```python
from build123d import *

# Parameters (mm, degrees)
SKETCH1_W                                            = 35
SKETCH1_H                                            = 38
BOSS_EXTRUDE1_DEPTH                                  = 4
M3_CLEARANCE_HOLE1_D                                 = 3.4
SKETCH4_R                                            = 11.05
CUT_EXTRUDE1_DEPTH                                   = 5
M3_CLEARANCE_HOLE2_D                                 = 3.4
CSK_FOR_M3_HEX_SOCKET_COUNTERSUNK_CAP_SC_D           = 3.4
CSK_FOR_M3_HEX_SOCKET_COUNTERSUNK_CAP_SC_CSINK_D     = 6.72
CSK_FOR_M3_HEX_SOCKET_COUNTERSUNK_CAP_SC_CSINK_ANGLE = 90
CSK_FOR_M3_HEX_SOCKET_COUNTERSUNK_CA_2_D             = 3.4
CSK_FOR_M3_HEX_SOCKET_COUNTERSUNK_CA_2_CSINK_D       = 6.72
CSK_FOR_M3_HEX_SOCKET_COUNTERSUNK_CA_2_CSINK_ANGLE   = 90


with BuildPart() as part:
    # Sketch1 → Boss-Extrude1 (new body)
    with BuildSketch(Plane(origin=(0, 0, 0), x_dir=(1, 0, 0), z_dir=(0, 1, 0))):
        Rectangle(SKETCH1_W, SKETCH1_H)
    extrude(amount=BOSS_EXTRUDE1_DEPTH)

    # M3 Clearance Hole1 (through all)
    with Locations(Plane(origin=(0, 0, 0), x_dir=(-1, 0, 0), z_dir=(0, -1, 0))):
        with Locations((-11.5, -13.5), (-11.5, 9.5), (11.5, 9.5), (11.5, -13.5)):
            Hole(M3_CLEARANCE_HOLE1_D / 2)

    # Sketch4 → Cut-Extrude1 (cut, through all)
    with BuildSketch(Plane(origin=(0, 4, 0), x_dir=(1, 0, 0), z_dir=(0, 1, 0))):
        with Locations((0, 1.5)):
            Circle(SKETCH4_R)
    extrude(amount=-CUT_EXTRUDE1_DEPTH, mode=Mode.SUBTRACT)

    # M3 Clearance Hole2 (through all)
    with Locations(Plane(origin=(0, 4, 0), x_dir=(1, 0, 0), z_dir=(0, 1, 0))):
        with Locations((-13, 14.5), (13, 14.5), (-13, -11.5), (13, -11.5)):
            Hole(M3_CLEARANCE_HOLE2_D / 2)

    # CSK for M3 Hex Socket Countersunk Cap Sc (through all)
    with Locations(Plane(origin=(0, 0, 0), x_dir=(-1, 0, 0), z_dir=(0, -1, 0))):
        with Locations((-13, 14.5), (13, 14.5)):
            CounterSinkHole(CSK_FOR_M3_HEX_SOCKET_COUNTERSUNK_CAP_SC_D / 2, CSK_FOR_M3_HEX_SOCKET_COUNTERSUNK_CAP_SC_CSINK_D / 2, counter_sink_angle=CSK_FOR_M3_HEX_SOCKET_COUNTERSUNK_CAP_SC_CSINK_ANGLE)

    # CSK for M3 Hex Socket Countersunk Ca 2 (through all)
    with Locations(Plane(origin=(0, 4, 0), x_dir=(1, 0, 0), z_dir=(0, 1, 0))):
        with Locations((11.5, 9.5), (-11.093205122, 9.5)):
            CounterSinkHole(CSK_FOR_M3_HEX_SOCKET_COUNTERSUNK_CA_2_D / 2, CSK_FOR_M3_HEX_SOCKET_COUNTERSUNK_CA_2_CSINK_D / 2, counter_sink_angle=CSK_FOR_M3_HEX_SOCKET_COUNTERSUNK_CA_2_CSINK_ANGLE)


solid = part.part
```
Geometry check sheet. Reference: the model listing, model coordinates, mm. A direction names the side the tool comes from. Round coordinates to 2 decimals unless told otherwise and drop trailing zeros. Loops run counter-clockwise (first coordinate to the right, second up) from the corner with the lowest first, then second, coordinate; pieces in that order, holes last. Notation, with made-up numbers: (-11.75, -1) - (14.25, -1) arc R22 ccw to (14.25, 33) - close; hole circle Ø10 at (-29, 9.25). An arc over 180 degrees is marked (long way). Write item = value, one per line. Start each with the question number.
1. Section check A-A on x = -7. Enter the section's corners in (y, z).
2. Thickness scan on line 1 (X direction, y = 3.2, z = -14.5); line 2 (Z direction, x = 13.5, y = 0.9); line 3 (Z direction, x = 13, y = 1.4). Record the ranges inside material, lowest first.
3. Section check D-D on y = 1.1. Enter the section's corners in (x, z).
4. Mould release check, pull along X, two halves, no side actions. Record for faces 1 (the face through (-13.8, 2.8, -13)), 2 (the face through (17.5, 2, 0)), 3 (the face through (-17.5, 2, 0)), 4 (the face through (0, 2, 19)): released by +X, released by -X, zero draft, split by the parting line, or undercut.
5. Section check C-C on z = -1.5. Enter the section's corners in (x, y).
6. Depth check by flat-ended pin: pin 1 (2.5 mm diameter, centred on x = 13, z = -14.5, fed in from -Y); pin 2 (5.5 mm diameter, centred on x = -11.09, z = -9.5, fed in from +Y); pin 3 (4 mm diameter, centred on x = -13, z = -14.5, fed in from -Y). Enter the tip coordinate at first touch or a pass-through.
7. Section check B-B on z = -14.5. Enter the section's corners in (x, y).
8. Set-up check for faces 5 (the face through (-8, 0, 8)), 6 (the face through (-13.2, 1.4, -9.5)): record each of +Z, -Z, +X, -X, +Y, -Y from which the full face is reachable in a straight line by a thin tool's end or side.
Working result:
q1.outline = (0, -19) - (4, -19) - (4, -10.05) - (0, -10.05) - close; (0, 7.05) - (4, 7.05) - (4, 19) - (0, 19) - close
q2.line_1 = -17.5 to -14.7, -11.3 to 11.3, 14.7 to 17.5
q2.line_2 = -19 to -16.91, -12.09 to 9.88, 13.12 to 19
q2.line_3 = -19 to -16.46, -12.54 to -10.3, -8.7 to 9.8, 14.3 to 19
q3.outline = (-17.5, -19) - (17.5, -19) - (17.5, 19) - (-17.5, 19) - close; hole circle Ø4.52 at (-13, -14.5); hole (-13.17, 13.19) arc R1.7 ccw (long way) to (-11.33, 11.81) arc R1.7 ccw (long way) to start; hole (-11.3, -11.19) arc R1.7 ccw (long way) to (-11.3, -7.81) arc R1.7 ccw (long way) to start; hole circle Ø22.1 at (0, -1.5); hole circle Ø3.4 at (11.5, -9.5); hole circle Ø4.52 at (13, -14.5); hole (11.33, 11.81) arc R1.7 ccw (long way) to (13.17, 13.19) arc R1.7 ccw (long way) to start
q4.face_1 = undercut
q4.face_2 = released by +X
q4.face_3 = released by -X
q4.face_4 = zero draft
q5.outline = (-17.5, 0) - (-11.05, 0) - (-11.05, 4) - (-17.5, 4) - close; (11.05, 0) - (17.5, 0) - (17.5, 4) - (11.05, 4) - close
q6.pin_1 = through
q6.pin_2 = 3.39
q6.pin_3 = 1.36
q7.outline = (-17.5, 0) - (-16.36, 0) - (-14.7, 1.66) - (-14.7, 4) - (-17.5, 4) - close; (-11.3, 1.66) - (-9.64, 0) - (9.64, 0) - (11.3, 1.66) - (11.3, 4) - (-11.3, 4) - close; (14.7, 1.66) - (16.36, 0) - (17.5, 0) - (17.5, 4) - (14.7, 4) - close
q8.face_5 = +Z, -Z, +X, -X, -Y
q8.face_6 = +Y, -Y
